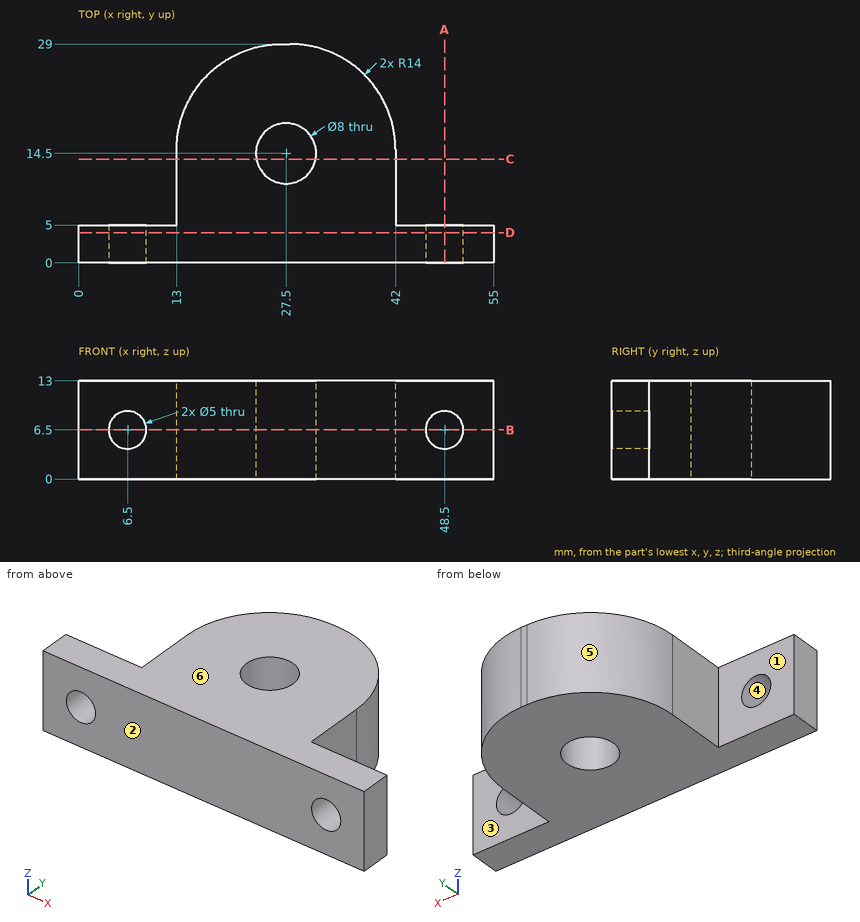
Part print with two shaded views. Sizes in mm from the minimum x, y, z corner. A direction names the side the tool comes from. Round coordinates to 2 decimals unless told otherwise and drop trailing zeros. Order: outer loops, then holes, each group sorted by start corner. A loop starts at its lowest first (then second) coordinate and runs counter-clockwise, first axis right, second up. Notation, with made-up numbers: (27.25, 75.25) -> (59.25, 75.25) arc R6 ccw to (59.25, 79.25) -> close; hole circle Ø11 at (88.25, 66). An arc over 180 degrees is marked (long way). Use one line per item in the form item = value.
Item 1: Drill centre lines: line 1 (Z direction, x = 48.5, y = 2.05); line 2 (X direction, y = 2.75, z = 6); line 3 (X direction, y = 14.75, z = 7.5). Where is each one in solid material? Low to high.
Returned:
line_1 = 0 to 4, 9 to 13
line_2 = 0 to 4.05, 8.95 to 46.05, 50.95 to 55
line_3 = 13 to 23.51, 31.49 to 42
Item 2: Cut at C-C, the plane y = 13.75. Write the cut outline in (x, z).
Returned:
outline = (13, 0) -> (23.57, 0) -> (23.57, 13) -> (13, 13) -> close; (31.43, 0) -> (42, 0) -> (42, 13) -> (31.43, 13) -> close
Item 3: Tool access for the marked faces 1, 2 and 3: list every direction of +Z, -Z, +X, -X, +Y, -Y with a clear straight run to the whole face (end or side of a thin tool).
Returned:
face_1 = +Z, -Z, -X, +Y
face_2 = +Z, -Z, +X, -X, -Y
face_3 = +Z, -Z, +X, +Y
Item 4: Cut at B-B, the plane z = 6.5. Write the cut outline in (x, y).
Returned:
outline = (0, 0) -> (4, 0) -> (4, 5) -> (0, 5) -> close; (9, 0) -> (46, 0) -> (46, 5) -> (42, 5) -> (42, 15) arc R14 ccw to (28, 29) -> (27, 29) arc R14 ccw to (13, 15) -> (13, 5) -> (9, 5) -> close; (51, 0) -> (55, 0) -> (55, 5) -> (51, 5) -> close; hole circle Ø8 at (27.5, 14.5)
Item 5: Cut at A-A, the plane x = 48.5. Write the cut outline in (y, z).
Returned:
outline = (0, 0) -> (5, 0) -> (5, 4) -> (0, 4) -> close; (0, 9) -> (5, 9) -> (5, 13) -> (0, 13) -> close
Item 6: Flat gauge pins, fed straight in: pin 1 Ø1.5 at (x, z) = (35, 6.5) entering from +Y; pin 2 Ø3 at (y, z) = (8.5, 11.5) entering from +X; pin 3 Ø4 at (x, z) = (35.5, 10) entering from +Y. Where does each tip first touch, or does it go through?
Returned:
pin_1 = 27.53
pin_2 = 42
pin_3 = 27.87
Item 7: Pull direction Z, two halves, no side cores. Call the marked faces 4, 5 and 6: released by +Z, released by -Z, zero draft, split by the parting line, or undercut.
Returned:
face_4 = undercut
face_5 = zero draft
face_6 = released by +Z
Item 8: Cut at D-D, the plane y = 4. Write the cut outline in (x, z).
Returned:
outline = (0, 0) -> (55, 0) -> (55, 13) -> (0, 13) -> close; hole circle Ø5 at (6.5, 6.5); hole circle Ø5 at (48.5, 6.5)
